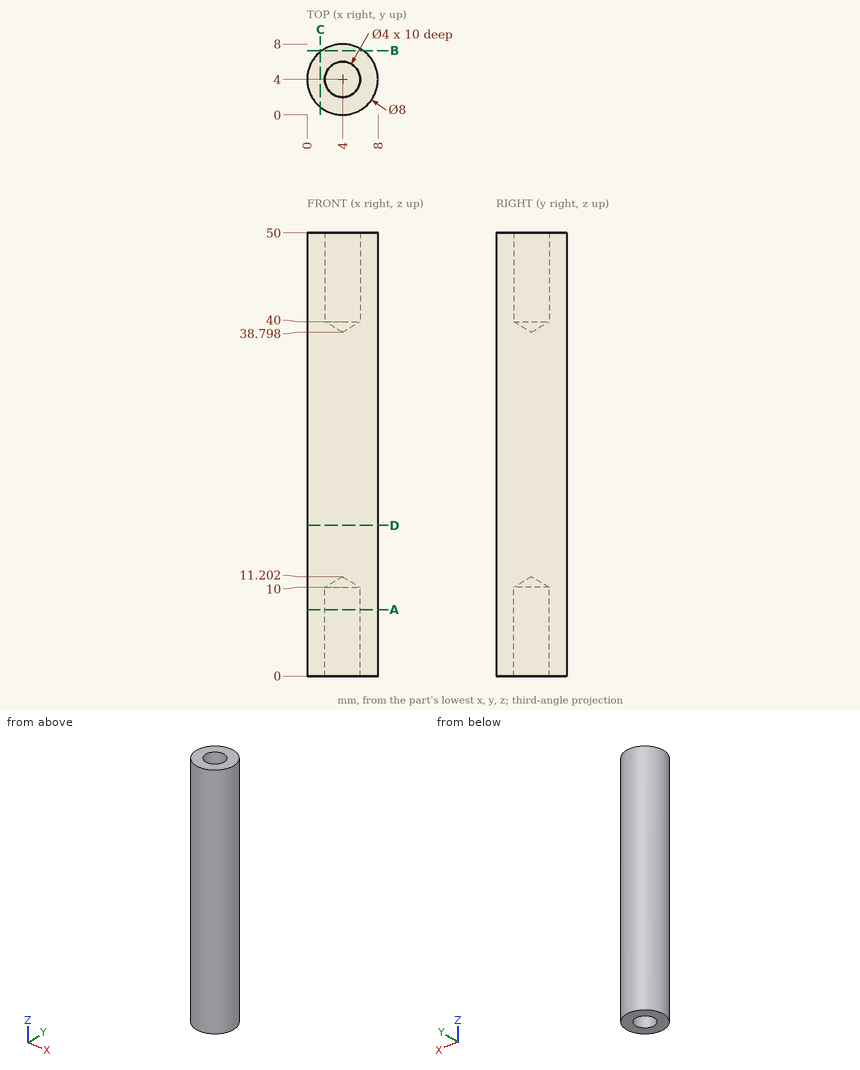
Here's the drawing with two shaded views (mm, measured from the low corner). I have some questions. Round coordinates to 2 decimals unless told otherwise and drop trailing zeros. Order: outer loops, then holes, each group sorted by start corner. A loop starts at its lowest first (then second) coordinate and runs counter-clockwise, first axis right, second up. Notation, with made-up numbers: (58, -21) -> (106, -21) arc R14 ccw to (106, -4) -> close; hole circle Ø10 at (22.25, -28.75). An arc over 180 degrees is marked (long way). Return JSON: item names as keys, results as strings.
Q1. I need wall thicknesses on line 1 along Y through (x, z) = (4, 48); line 2 along Y through (x, z) = (3.75, 17); line 3 along X through (y, z) = (3, 33). Which ranges of each line are inside material? Lowest first, please. Write a range as from..to.
Filled sheet:
{"line 1": "y = 0..2, 6..8", "line 2": "y = 0.01..7.99", "line 3": "x = 0.13..7.87"}
Q2. For pin 1 Ø3.5 at (x, y) = (4, 4) entering from -Z, with a flat end and sliding along its axis, tell me the tip position at first contact or that it passes through.
Filled sheet:
{"pin 1": "stops at z = 10.15"}
Q3. If we section it at D-D on z = 17: List the corners of the cut face in (x, y) for me, plus the area to 3 significant figures.
Filled sheet:
{"outline": "circle Ø8 at (4, 4)", "area": "50.3 mm^2"}
Q4. If we section it at A-A on z = 7.5: List the corners of the cut face in (x, y) for me, plus the area to 3 significant figures.
Filled sheet:
{"outline": "circle Ø8 at (4, 4); hole circle Ø4 at (4, 4)", "area": "37.7 mm^2"}
Q5. If we section it at C-C on x = 1.5: List the corners of the cut face in (y, z) for me.
Filled sheet:
{"outline": "(0.88, 0) -> (7.12, 0) -> (7.12, 50) -> (0.88, 50) -> close"}
Q6. If we section it at B-B on y = 7.25: List the corners of the cut face in (x, z) for me, plus the area to 3 significant figures.
Filled sheet:
{"outline": "(1.67, 0) -> (6.33, 0) -> (6.33, 50) -> (1.67, 50) -> close", "area": "233 mm^2"}
